Model file for the job. Use its own axes, mm. Coordinates: 2 decimals unless noted, no trailing zeros. Write each loop counter-clockwise with the first axis right and the second up, starting at its lowest first coordinate (ties: lowest second). Pieces come first, ordered by that corner, then holes. Notation, with made-up numbers: M 54,57 L 88,57 A20 cw 88,68 Z; hole C 22,3.25 d6. An arc over 180 degrees is marked long. Answer in a Markdown table with one row per item. Add a question column.
Autodesk Inventor part; units mm, degrees
ref_plane "YZ Plane" through (0, 0, 0) normal (1, 0, 0) x (0, 1, 0)
ref_plane "XZ Plane" through (0, 0, 0) normal (0, 1, 0) x (-1, 0, 0)
ref_plane "XY Plane" through (0, 0, 0) normal (0, 0, 1) x (1, 0, 0)
sketch "Sketch1" plane through (0, 0, 0) normal (0, 0, 1) x (1, 0, 0)
  line L0 (-11.5, -17.5) -> (11.5, -17.5)
  line L1 (11.5, -17.5) -> (11.5, 17.5)
  line L2 (11.5, 17.5) -> (-11.5, 17.5)
  line L3 (-11.5, 17.5) -> (-11.5, -17.5)
  line L4 (-11.5, -17.5) -> (11.5, 17.5) construction
  line L5 (11.5, -17.5) -> (-11.5, 17.5) construction
  point P0 (0, 0)
  dimension "d0" = 23
  dimension "d1" = 35
extrude "Plate1" add sketch "Sketch1" along normal blind 1
sketch "Sketch2" plane through (0, 0, 1) normal (0, 0, 1) x (1, 0, 0)
  line L0 (-11.5, -17.5) -> (-11.5, 17.5)
  point P0 (0, 0)
  point P1 (-9, -13)
  point P2 (9, -13)
  point P3 (-9, -5)
  point P4 (9, -5)
  dimension "d3" = 18
  dimension "d4" = 9
  dimension "d5" = 8
  dimension "d8" = 2.5
  dimension "d17" = 5
hole "Hole1" at (-9, -13, 1) at (9, -13, 1) at (-9, -5, 1) at (9, -5, 1) direction (0, 0, -1) diameter 2.5 depth 1
fillet "Fillet1" radius 2.5 4 edges at (11.5, 17.5, 0.5) (11.5, -17.5, 0.5) (-11.5, -17.5, 0.5) (-11.5, 17.5, 0.5)
mirror "Mirror1" about plane through (0, 0, 0) normal (0, 1, 0) of "Hole1"
equation "\"d14\" = Stärke"
equation "\"d2\" = Stärke"
equation "\"Biegeradius\" = Stärke"
equation "\"BreiteBiegungsfreistellung\" = Stärke"
equation "\"TiefeBiegungsfreistellung\" = 0.5 * Stärke"
equation "\"GrößeEckenfreistellung\" = 4 * Stärke"
equation "\"MinimalRest\" = 2 * Stärke"
equation "\"Übergangsradius\" = Biegeradius"
equation "\"JacobiRadiusGröße\" = Biegeradius"
equation "\"Abstandsgröße\" = Stärke"
properties part number "17"
1) Drill centre lines: probe 1 along X at (y, z) = (5, 0.3); probe 2 along Y at (x, z) = (-9, 0.7); probe 3 along X at (y, z) = (16, 0.4). Where is each one in solid material? Low to high.
2) Slice it at A-A (y = 13). Give the cut face in (x, z).
3) Slice it at B-B (z = 0.6). Count the separate pieces of the cut face and the enclosed holes in it, then the cut area to 3 significant figures.
Ans:
| question | item | result |
|---|---|---|
| 1 | probe 1 | x = -11.5 to -10.25, -7.75 to 7.75, 10.25 to 11.5 |
| 1 | probe 2 | y = -17.5 to -14.25, -11.75 to -6.25, -3.75 to 3.75, 6.25 to 11.75, 14.25 to 17.5 |
| 1 | probe 3 | x = -11.29 to 11.29 |
| 2 | outline | M -11.5,0 L -10.25,0 L -10.25,1 L -11.5,1 Z; M -7.75,0 L 7.75,0 L 7.75,1 L -7.75,1 Z; M 10.25,0 L 11.5,0 L 11.5,1 L 10.25,1 Z |
| 3 | separate pieces | 1 |
| 3 | enclosed holes | 8 |
| 3 | area | 760 mm2 |
